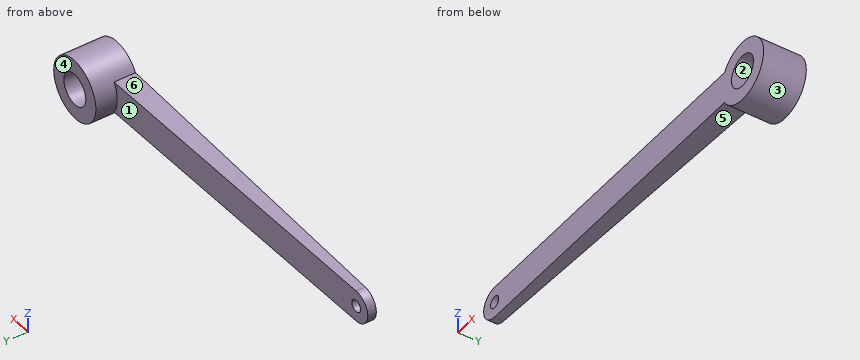
from build123d import *

# Parameters (mm, degrees)
SKETCH1_R               = 9.144
SKETCH1_R_2             = 4.7625
BOSS_EXTRUDE1_DEPTH     = 12.7
SKETCH2_R               = 1.778
BOSS_EXTRUDE2_DEPTH     = 6.35
SKETCH3_R               = 4.7625
CUT_EXTRUDE1_DEPTH      = 13.97
CUT_EXTRUDE3_DEPTH      = 10.144
CUT_EXTRUDE3_DEPTH_BACK = 10.144


with BuildPart() as part:
    # Sketch1 → Boss-Extrude1 (new body)
    with BuildSketch(Plane(origin=(0, 0, 0), x_dir=(1, 0, 0), z_dir=(0, 1, 0))):
        Circle(SKETCH1_R)
        Circle(SKETCH1_R_2, mode=Mode.SUBTRACT)
    extrude(amount=BOSS_EXTRUDE1_DEPTH)

    # Sketch2 → Boss-Extrude2 (add)
    with BuildSketch(Plane(origin=(0, 0, 0), x_dir=(1, 0, 0), z_dir=(0, 1, 0))):
        with BuildLine():
            Line((0, -4.7625), (0, 4.7625))
            Line((0, 4.7625), (-107.442, 4.7625))
            ThreePointArc((-107.442, 4.7625), (-112.2045, 0), (-107.442, -4.7625))
            Line((-107.442, -4.7625), (0, -4.7625))
        make_face()
        with Locations((-107.442, 0)):
            Circle(SKETCH2_R, mode=Mode.SUBTRACT)
    extrude(amount=BOSS_EXTRUDE2_DEPTH)

    # Sketch3 → Cut-Extrude1 (cut)
    with BuildSketch(Plane(origin=(0, 12.7, 0), x_dir=(1, 0, 0), z_dir=(0, 1, 0))):
        Circle(SKETCH3_R)
    extrude(amount=-CUT_EXTRUDE1_DEPTH, mode=Mode.SUBTRACT)

    # Sketch4 → Cut-Extrude3 (cut, two sides)
    with BuildSketch(Plane.XY) as cut_extrude3_sk:
        Polygon((-112.2045, 2.54), (-112.2045, 6.35), (-9.144, 6.35), align=None)
    extrude(amount=CUT_EXTRUDE3_DEPTH, mode=Mode.SUBTRACT)
    extrude(cut_extrude3_sk.sketch, amount=-CUT_EXTRUDE3_DEPTH_BACK, mode=Mode.SUBTRACT)


solid = part.part
Source: CAD feature listing. Evaluate the final solid. Frame: model axes, mm. Face numbers are marked on the shaded views. A direction names the side the tool comes from. Give positions to 0.01 mm unless a question says otherwise; leave off trailing zeros. Loops run counter-clockwise (first coordinate to the right, second up) from the corner with the lowest first, then second, coordinate; pieces in that order, holes last. Notation, with made-up numbers: (-31.75, 82.5) -> (-1.75, 82.5) arc R24 cw to (-1.75, 110.5) -> close; hole circle Ø2 at (6, -14.5). An arc over 180 degrees is marked (long way). Use a Markdown table: item, result. Add a question column.
1) Section query C-C, the plane y = 4.5. Return the cut outline in (x, z) (1 decimal).
2) Pull-direction query (Z, two-part tool) for the marked faces 1, 2 and 3; classes: +Z half, -Z half, draft (parallel to the pull), parting line (faces both ways), or undercut.
3) First-contact query: pin 1 (1.5 mm diameter, centred on x = -72, y = 3, fed in from +Z); pin 2 (6 mm diameter, centred on x = -78, z = 4.5, fed in from +Y); pin 3 (1.9 mm diameter, centred on x = -70, y = 4, fed in from -Z). Flat tips, straight axial feed; report the tip coordinate or a pass-through.
4) Section query A-A, the plane x = 0. Return the cut outline in (y, z), then the cut area to 3 significant figures.
5) Reachability of the marked faces 4, 5 and 6 from +Z, -Z, +X, -X, +Y, -Y: full face, straight path, thin tool, end or side. Return the list, or none.
6) Section query B-B, the plane z = -3.75. Return the cut outline in (x, y).
7) Line query: line 1 along X through (y, z) = (9, 0); line 2 along X through (y, z) = (7.75, 4.25). Output: solid intervals per line, ascending. Write a range as [from, to].
8) Section query D-D, the plane z = 3. Return the cut outline in (x, y).
Numbers:
| question | item | result |
|---|---|---|
| 1 | outline | (-59.2, -4.8) -> (-7.8, -4.8) arc R9.1 ccw (long way) to (-7.8, 4.8) -> (-59.2, 4.8) -> close; hole circle Ø9.5 at (0, 0) |
| 2 | face 1 | draft |
| 2 | face 2 | undercut |
| 2 | face 3 | parting line |
| 3 | pin 1 | stops at z = 4.76 |
| 3 | pin 2 | stops at y = 3.92 |
| 3 | pin 3 | stops at z = -4.76 |
| 4 | outline | (0, -9.14) -> (12.7, -9.14) -> (12.7, -4.76) -> (0, -4.76) -> close; (0, 4.76) -> (12.7, 4.76) -> (12.7, 9.14) -> (0, 9.14) -> close |
| 4 | area | 111 mm2 |
| 5 | face 4 | +Z, -Z, +X, -X, +Y |
| 5 | face 5 | -Z, -X, +Y, -Y |
| 5 | face 6 | +Z, -X, +Y, -Y |
| 6 | outline | (-110.38, 0) -> (-2.94, 0) -> (-2.94, 12.7) -> (-8.34, 12.7) -> (-8.34, 6.35) -> (-9.14, 6.35) -> (-110.38, 2.61) -> close; (2.94, 0) -> (8.34, 0) -> (8.34, 12.7) -> (2.94, 12.7) -> close |
| 7 | line 1 | x = [-9.14, -4.76], [4.76, 9.14] |
| 7 | line 2 | x = [-8.1, -2.15], [2.15, 8.1] |
| 8 | outline | (-111.14, 0) -> (-3.7, 0) -> (-3.7, 12.7) -> (-8.64, 12.7) -> (-8.64, 6.35) -> (-9.14, 6.35) -> (-111.14, 2.58) -> close; (3.7, 0) -> (8.64, 0) -> (8.64, 12.7) -> (3.7, 12.7) -> close |
